```python
from build123d import *

# Parameters (mm, degrees)
BOSS_EXTRUDE1_DEPTH     = 17
CUT_EXTRUDE1_DEPTH      = 15
CUT_EXTRUDE2_DEPTH      = 46.197309304
CUT_EXTRUDE2_DEPTH_BACK = 46.197309304
CUT_EXTRUDE3_DEPTH      = 12
SKETCH6_R               = 4
CUT_EXTRUDE4_DEPTH      = 35
CUT_EXTRUDE5_START      = -12.78511231
CUT_EXTRUDE5_OUTLINE_W  = 3.3
CUT_EXTRUDE5_OUTLINE_H  = 13.870481222
CUT_EXTRUDE5_DEPTH      = 12.78511231
SKETCH8_R               = 1.25
CUT_EXTRUDE6_DEPTH      = 15
SKETCH10_R              = 1.25
CUT_EXTRUDE7_DEPTH      = 15
FILLET1_SIZE            = 2
FILLET1_SIZE_2          = 10


# Read off the part's stored shape, not the designer's step: Cut-Extrude5, Extrude-Thin1
with BuildPart() as part:
    # Sketch1 → Boss-Extrude1 (new body)
    with BuildSketch(Plane.XY):
        Polygon((-9.564728379, 17.62000192), (-5.473819301, 18.015682238), (-6.704675095, 30.741407789), (2.153984466, 31.598233783), (3.38531081, 18.867643246), (7.473335954, 19.262913811), (8.876277245, 4.753208867), (22.578615379, 5.119591375), (30.743737203, -1.458779689), (27.230396467, -5.819563663), (20.33101325, -0.260956714), (8.140408694, -15.392023407), (15.036201119, -20.947737373), (11.522860383, -25.308521347), (3.283942394, -18.670695131), (-7.860727511, 0), align=None)
    extrude(amount=BOSS_EXTRUDE1_DEPTH)

    # Sketch3 → Cut-Extrude1 (cut)
    with BuildSketch(Plane(origin=(-3.696725775, -0.357554178, 0), x_dir=(0, 0, 1), z_dir=(-0.9953550068413657, -0.09627258361457379, 0))):
        with BuildLine():
            Line((0, 31.244090554), (0, 32.721435634))
            Line((0, 32.721435634), (17.68, 32.721435634))
            Line((17.68, 32.721435634), (17.68, 18.458978244))
            Line((17.68, 18.458978244), (14.22, 18.458978244))
            Line((14.22, 18.458978244), (16.043166109, 22.04177957))
            ThreePointArc((16.043166109, 22.04177957), (15.680947079, 27.433223117), (11.85, 31.244090554))
            Line((11.85, 31.244090554), (0, 31.244090554))
        make_face()
    extrude(amount=-CUT_EXTRUDE1_DEPTH, mode=Mode.SUBTRACT)

    # Sketch4 → Cut-Extrude2 (cut, two sides: drawn at the far end of the back side and taken through both)
    with BuildSketch(Plane(origin=(7.87496966, 9.774469394, 0), x_dir=(0.7787114240648987, -0.6273822742402098, 0), z_dir=(-0.6273822742402096, -0.7787114240648986, 0)).offset(-CUT_EXTRUDE2_DEPTH_BACK)):
        Polygon((15.990906633, 19.904885529), (15.990906633, 16.999999998), (15.995711897, 16.999999998), (23.069210216, 16.999999998), (24.855711897, 17), (24.855711897, 0), (20.721010741, 0), (15.995711897, -2e-09), (15.990906633, -2e-09), (15.990906633, -2.308790515), (29.141254547, -2.308790515), (29.141254547, 19.904885529), align=None)
        with BuildLine():
            Line((24.855711897, 17), (23.069210216, 17))
            Line((23.069210216, 16.999999998), (23.069210216, 13.096000073))
            ThreePointArc((23.069210216, 13.096000073), (24.441573822, 8.347001118), (23.069216362, 3.598000386))
            add(Edge.make_bspline(
                [(20.721010741, -2e-09), (22.390075827, 1.367964254), (23.069216362, 3.598000386)],
                knots=[0, 0, 0, 1, 1, 1], degree=2))
            Line((20.721010741, 0), (24.855711897, 0))
            Line((24.855711897, 0), (24.855711897, 17))
        make_face()
    extrude(amount=CUT_EXTRUDE2_DEPTH + CUT_EXTRUDE2_DEPTH_BACK, mode=Mode.SUBTRACT)

    # Sketch5 → Cut-Extrude3 (cut)
    with BuildSketch(Plane(origin=(-4.315634896, -5.356597299, 0), x_dir=(0.7787114240649037, -0.6273822742402033, 0), z_dir=(0.6273822742402033, 0.7787114240649037, 0))):
        with BuildLine():
            Line((15.990245326, -16.999999999), (23.069210216, -16.999999999))
            Line((23.069210216, -16.999999999), (23.069210216, -13.096000073))
            ThreePointArc((23.069210216, -13.096000073), (20.032304179, -15.959301473), (15.990245326, -16.999999999))
        make_face()
    extrude(amount=-CUT_EXTRUDE3_DEPTH, mode=Mode.SUBTRACT)

    # Sketch6 → Cut-Extrude4 (cut)
    with BuildSketch(Plane(origin=(11.388310395, 14.135253369, 0), x_dir=(0.7787114240649039, -0.6273822742402033, 0), z_dir=(0.6273822742402032, 0.7787114240649039, 0))):
        with Locations(Location((19.069210216, -8.499999999, 0), (0, 0, 180))):
            Circle(SKETCH6_R)
    extrude(amount=-CUT_EXTRUDE4_DEPTH, mode=Mode.SUBTRACT)

    # Cut-Extrude5 outline → Cut-Extrude5 (cut)
    with BuildSketch(Plane(origin=(-3.00794932, 31.098961967, 0), x_dir=(0.995355006841366, 0.0962725836145697, 0), z_dir=(-0.0962725836145697, 0.995355006841366, 0)).offset(CUT_EXTRUDE5_START)):
        with Locations((0.736022827, -9.435240611)):
            Rectangle(CUT_EXTRUDE5_OUTLINE_W, CUT_EXTRUDE5_OUTLINE_H)
    extrude(amount=CUT_EXTRUDE5_DEPTH, mode=Mode.SUBTRACT)

    # Sketch8 → Cut-Extrude6 (cut)
    with BuildSketch(Plane(origin=(5.161933786, 0.499271816, 0), x_dir=(0, 0, -1), z_dir=(0.9953550068413664, 0.09627258361456668, 0))):
        with Locations(Location((-8.8, 27.244090554, 0), (0, 0, 90))):
            Circle(SKETCH8_R)
    extrude(amount=-CUT_EXTRUDE6_DEPTH, mode=Mode.SUBTRACT)

    # Extrude-Thin1 outline → Extrude-Thin1 (revolve)
    with BuildSketch(Plane(origin=(-2.622858986, 27.11754194, 8.8), x_dir=(-0.0962725836145697, 0.9953550068413659, 0), z_dir=(0, 0, -1))):
        Polygon((1.25, 0.736022827), (0.297372056, -0.913977173), (3.202627944, -0.913977173), (2.25, 0.736022827), (3.202627944, 2.386022827), (0.297372056, 2.386022827), align=None)
    revolve(axis=Axis((-2.622858986, 27.11754194, 8.8), (0.9953550068413659, 0.0962725836145697, 0)))

    # Sketch10 → Cut-Extrude7 (cut)
    with BuildSketch(Plane(origin=(5.161933786, 0.499271816, 0), x_dir=(0, 0, -1), z_dir=(0.9953550068413664, 0.09627258361456668, 0))):
        with Locations(Location((-8.8, 27.244090554, 0), (0, 0, 90))):
            Circle(SKETCH10_R)
    extrude(amount=-CUT_EXTRUDE7_DEPTH, mode=Mode.SUBTRACT)

    # Fillet1
    # an asymmetric fillet: 10, 2 mm, written as the material it takes off along each edge
    with BuildSketch(Plane(origin=(-31.588550266, 28.334593199, 0), x_dir=(0, 0, 1), z_dir=(0.995355006841366, 0.0962725836145696, 0))) as fillet1_piece_1:
        with BuildLine():
            Bezier((FILLET1_SIZE, 0), (0, 0), (0, FILLET1_SIZE_2), weights=[1, 0.707106781, 1])
            Line((0, FILLET1_SIZE_2), (0, 0))
            Line((0, 0), (FILLET1_SIZE, 0))
        make_face()
    extrude(amount=58.9, mode=Mode.SUBTRACT)


solid = part.part
```
The model under review builds one solid part; all positions refer to its coordinate system, in mm. A direction names the side the tool comes from. Round coordinates to 2 decimals unless told otherwise and drop trailing zeros. Loops run counter-clockwise (first coordinate to the right, second up) from the corner with the lowest first, then second, coordinate; pieces in that order, holes last. Notation, with made-up numbers: (79, -8) -> (103, -8) arc R26 ccw to (103, 9) -> close; hole circle Ø5 at (42, -18.5). An arc over 180 degrees is marked (long way). Answer as a JSON object with one key per item and string values. Group by question number.
1) We need section A-A on y = 26.5. Give the number of separate pieces and of enclosed holes in the cut face, then the cut area to 3 significant figures.
2) Mouldability with a two-part tool opening along X and no side actions: class faces 1 (the face through (5, 0, 0)), 2 (the face through (13.575, -19.771, 6.492)), 3 (the face through (-4.27, 19.91, 15.12)), 4 (the face through (3.78, -19.07, 8.38)) as released by +X, released by -X, zero draft, split by the parting line, or undercut.
3) For faces 5 (the face through (14.32, -7.72, 2.93)), 6 (the face through (-2, 25, 2.5)), 7 (the face through (1.11, 27.6, 15.71)), 8 (the face through (5.401, 19.063, 8.381)), 9 (the face through (27.62, -2.49, 15.08)), list the 3-axis set-ups (+Z, -Z, +X, -X, +Y, -Y) from which the entire face can be reached by the end or side of a thin tool; tool diameter is ignored.
4) We need section B-B on y = 16.5. Write out the cut boundary in (x, z).
5) For pin 1 Ø3.5 at (x, y) = (-1, 25) entering from +Z; pin 2 Ø2 at (x, z) = (0.5, 5) entering from -Y; pin 3 Ø4 at (x, z) = (20, 3) entering from +Y, all flat-tipped, find the tip position at first contact; note any pin that passes through.
6) For line 1 (Y direction, x = -1.5, z = 9.75); line 2 (Z direction, x = 28.5, y = -0.5); line 3 (X direction, y = -4.5, z = 3.25), list the stretches that pass through material, from the lowest coordinate up. Write a range as [from, to].
7) We need section C-C on y = 8. Write out the cut boundary in (x, z).
Result set:
{
 "1": {"separate pieces": "2", "enclosed holes": "1", "area": "95.3 mm²"},
 "2": {"face 1": "zero draft", "face 2": "released by +X", "face 3": "undercut", "face 4": "released by -X"},
 "3": {"face 5": "+Z, -Z", "face 6": "none", "face 7": "+Z", "face 8": "+Z, -Z, +Y", "face 9": "+Z, +X, -Y"},
 "4": {"outline": "(-9.46, 0) -> (7.74, 0) -> (7.74, 17) -> (-9.46, 17) -> close"},
 "5": {"pin 1": "z = 16.37", "pin 2": "y = -15.68", "pin 3": "y = 5.1"},
 "6": {"line 1": "[-10.66, 18.4], [25.06, 26.41], [28.04, 29.67]", "line 2": "[2.21, 6.46], [10.54, 17]", "line 3": "[-5.17, 16.92], [25.59, 25.85]"},
 "7": {"outline": "(-8.63, 0) -> (8.56, 0) -> (8.56, 17) -> (-8.63, 17) -> close"}
}
